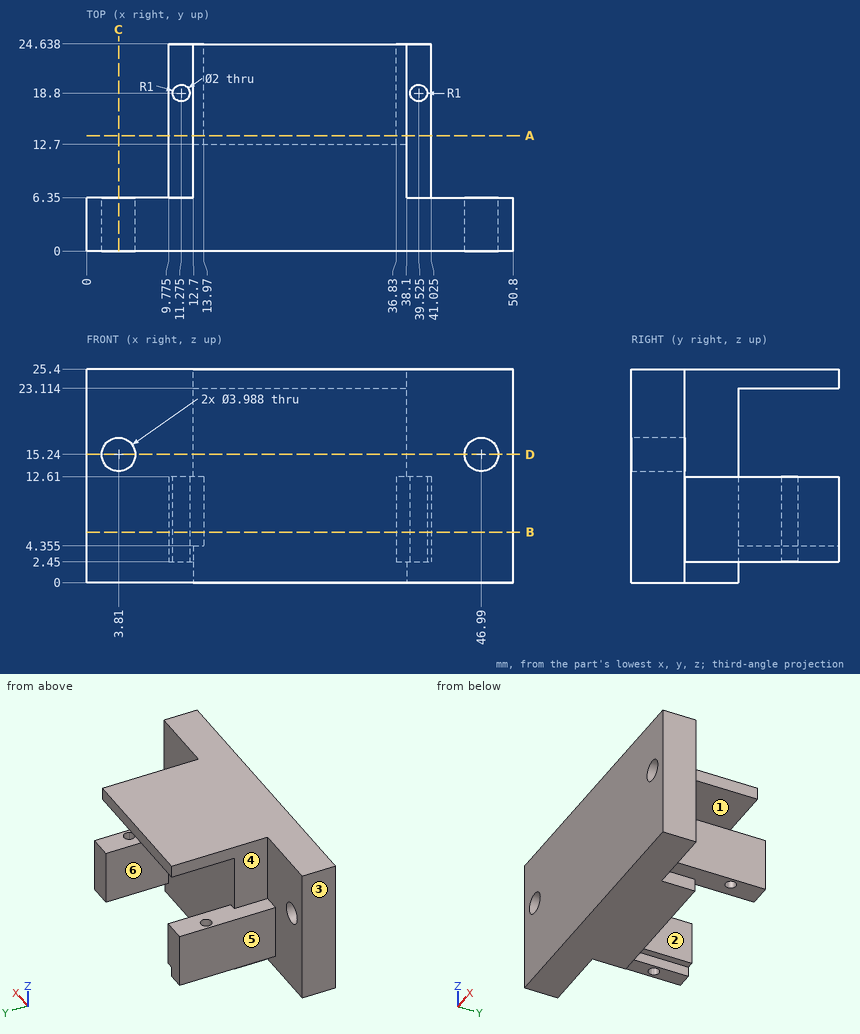
For this review, use the dimensioned drawing (mm, ordinates from the lowest corner) and the shaded views. A direction names the side the tool comes from. Round coordinates to 2 decimals unless told otherwise and drop trailing zeros. Write each loop counter-clockwise with the first axis right and the second up, starting at its lowest first coordinate (ties: lowest second). Pieces come first, ordered by that corner, then holes. Notation, with made-up numbers: (78, 58) -> (128, 58) arc R19 ccw to (128, 69) -> close; hole circle Ø8 at (80.5, -33.5). An arc over 180 degrees is marked (long way). Use CSV: the item, a comma, the result in double quotes.
Q1. Consider section D-D (z = 15.24). Give the boundary of the cut face in (x, y).
Checks:
outline,"(0, 0) -> (1.82, 0) -> (1.82, 6.35) -> (0, 6.35) -> close; (5.8, 0) -> (45, 0) -> (45, 6.35) -> (38.1, 6.35) -> (38.1, 12.7) -> (12.7, 12.7) -> (12.7, 6.35) -> (5.8, 6.35) -> close; (48.98, 0) -> (50.8, 0) -> (50.8, 6.35) -> (48.98, 6.35) -> close"
Q2. For the marked faces 4, 5 and 6, list the 3-axis set-ups (+Z, -Z, +X, -X, +Y, -Y) from which the entire face can be reached by the end or side of a thin tool; tool diameter is ignored.
Checks:
face 4,"+Z, -X, +Y"
face 5,"+Z, -Z, -X, +Y"
face 6,"-Z, +Y"
Q3. For pin 1 Ø0.9 at (x, y) = (11, 11.5) entering from -Z; pin 2 Ø4 at (x, z) = (7.5, 13) entering from +Y; pin 3 Ø2 at (x, y) = (40, 13) entering from +Z, all flat-tipped, find the tip position at first contact; note any pin that passes through.
Checks:
pin 1,"z = 2.45"
pin 2,"y = 6.35"
pin 3,"z = 12.61"
Q4. Consider section B-B (z = 6). Give the boundary of the cut face in (x, y) (3 decimals).
Checks:
outline,"(0, 0) -> (50.8, 0) -> (50.8, 6.35) -> (41.025, 6.35) -> (41.025, 24.638) -> (36.83, 24.638) -> (36.83, 12.7) -> (13.97, 12.7) -> (13.97, 24.638) -> (9.775, 24.638) -> (9.775, 6.35) -> (0, 6.35) -> close; hole circle Ø2 at (11.275, 18.8); hole circle Ø2 at (39.525, 18.8)"
Q5. Mouldability with a two-part tool opening along X and no side actions: class the marked faces 1, 2 and 3 as released by +X, released by -X, zero draft, split by the parting line, or undercut.
Checks:
face 1,"zero draft"
face 2,"undercut"
face 3,"released by -X"
Q6. Consider section C-C (x = 3.81). Give the boundary of the cut face in (y, z), then the cut area to 3 significant figures.
Checks:
outline,"(0, 0) -> (6.35, 0) -> (6.35, 13.25) -> (0, 13.25) -> close; (0, 17.23) -> (6.35, 17.23) -> (6.35, 25.4) -> (0, 25.4) -> close"
area,"136 mm²"
Q7. Consider section A-A (y = 13.75). Give the boundary of the cut face in (x, z) (3 decimals), then the cut area to 3 significant figures.
Checks:
outline,"(9.775, 2.45) -> (12.7, 2.45) -> (12.7, 4.355) -> (13.97, 4.355) -> (13.97, 12.61) -> (9.775, 12.61) -> close; (12.7, 23.114) -> (38.1, 23.114) -> (38.1, 25.4) -> (12.7, 25.4) -> close; (36.83, 2.45) -> (41.025, 2.45) -> (41.025, 12.61) -> (36.83, 12.61) -> close"
area,"141 mm²"
Q8. To check wall thickness, follow probe 1 along X at (y, z) = (4.25, 15.24); probe 2 along X at (y, z) = (18.8, 7.75) (3 decimals); probe 3 along Z at (x, y) = (46.99, 4.5). State the ranges of each line that lie inside material, in increasing order. Write a range as [from, to].
Checks:
probe 1,"[0, 1.82], [5.8, 45], [48.98, 50.8]"
probe 2,"[9.775, 10.275], [12.275, 13.97], [36.83, 38.525], [40.525, 41.025]"
probe 3,"[0, 13.25], [17.23, 25.4]"
